Answer from the drawing. Dimensions are ordinates in mm from the lowest x, y and z of the part. A direction names the side the tool comes from. Give positions to 0.01 mm unless a question says otherwise; leave off trailing zeros. Loops run counter-clockwise (first coordinate to the right, second up) from the corner with the lowest first, then second, coordinate; pieces in that order, holes last. Notation, with made-up numbers: (66.25, -14.75) -> (86.25, -14.75) arc R19 ccw to (86.25, 2.25) -> close; hole circle Ø1 at (-22.75, 2). An arc over 180 degrees is marked (long way). Write each question's results on one line, items separated by ' | '. Start each with the question number.
Item 1: Section B-B on y = 20 is taken. Write down the section's boundary in (x, z).
Item 2: Section D-D on y = 7.5 is taken. Write down the section's boundary in (x, z), and give its area (3 significant figures).
Item 3: Which of the six approach directions +Z, -Z, +X, -X, +Y, -Y give full straight-line access (tool end or side, diameter ignored) to the marked faces 1 and 2?
Item 4: Section A-A on z = 18.5 is taken. Write down the section's boundary in (x, y).
Item 5: Find the intervals of material crossed by line 1 (Y direction, x = 30, z = 39); line 2 (Z direction, x = 8, y = 15.5); line 3 (X direction, y = 4.5, z = 6), in increasing order.
Item 6: Each of these flat-tipped pins is pushed along its axis until it touches: P1, Ø2.5, axis at y = 29, z = 9.5, coming from the -X side; P2, Ø8, axis at x = 11.5, y = 9.5, coming from the -Z side; P3, Ø6, axis at y = 11, z = 32, coming from the +X side. Where does it stop, or does it pass through?
Item 7: Section C-C on x = 30 is taken. Write down the section's boundary in (y, z).
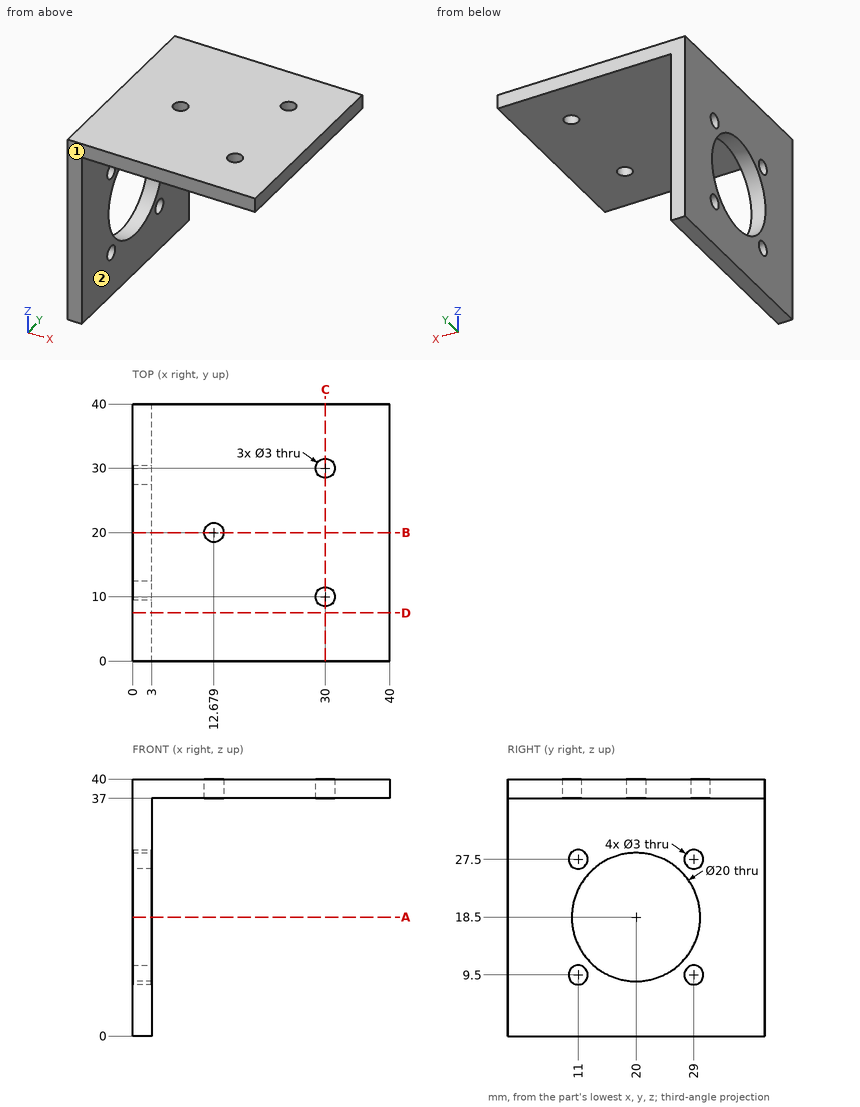
Findings:
1) outline: (0, 0) -> (3, 0) -> (3, 8.5) -> (0, 8.5) -> close; (0, 28.5) -> (3, 28.5) -> (3, 37) -> (11.18, 37) -> (11.18, 40) -> (0, 40) -> close; (14.18, 37) -> (40, 37) -> (40, 40) -> (14.18, 40) -> close
2) outline: (0, 0) -> (3, 0) -> (3, 37) -> (40, 37) -> (40, 40) -> (0, 40) -> close | area: 231 mm2
3) face 1: +Z, -Z, +X, -X, -Y | face 2: -Z, +X, +Y, -Y
4) outline: (0, 0) -> (3, 0) -> (3, 10) -> (0, 10) -> close; (0, 30) -> (3, 30) -> (3, 40) -> (0, 40) -> close
5) line 1: 0 to 8.5, 11.5 to 28.5, 31.5 to 40 | line 2: 37 to 40 | line 3: 0 to 3
6) P1: through | P2: z = 37 | P3: x = 3
7) outline: (0, 37) -> (8.5, 37) -> (8.5, 40) -> (0, 40) -> close; (11.5, 37) -> (28.5, 37) -> (28.5, 40) -> (11.5, 40) -> close; (31.5, 37) -> (40, 37) -> (40, 40) -> (31.5, 40) -> close
